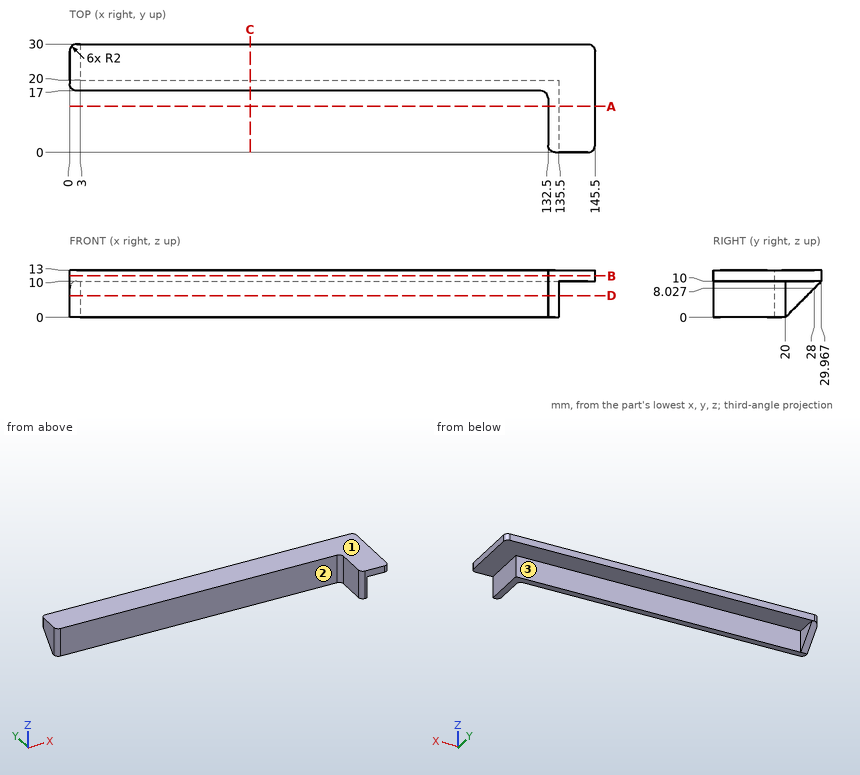
Input: dimensioned drawing with shaded views. Units: mm. Origin: part minimum x, y, z. A direction names the side the tool comes from. Round coordinates to 2 decimals unless told otherwise and drop trailing zeros. Order: outer loops, then holes, each group sorted by start corner. A loop starts at its lowest first (then second) coordinate and runs counter-clockwise, first axis right, second up. Notation, with made-up numbers: (35.5, 5.5) - (85.5, 5.5) arc R26 cw to (85.5, 44.5) - close; hole circle Ø8 at (-25, 1). An arc over 180 degrees is marked (long way). Answer as a JSON object with one key per item and string values. Group by question number.
(1) Cut plane D-D (z = 6). Return loops of the section in (x, y).
(2) Cut plane B-B (z = 11.5). Return loops of the section in (x, y).
(3) Pin query (flat end, axial travel): P1, Ø5, axis at y = 24, z = 4.5, coming from the +X side; P2, Ø4, axis at y = 12.5, z = 11, coming from the -X side; P3, Ø4, axis at x = 94.5, y = 16.5, coming from the +Z side; P4, Ø4, axis at y = 13, z = 7, coming from the +X side. Return the tip coordinate at first contact, or that it passes through.
(4) Reachability of the marked faces 1, 2 and 3 from +Z, -Z, +X, -X, +Y, -Y: full face, straight path, thin tool, end or side. Return the list, or none.
(5) Cut plane A-A (y = 12.75). Return loops of the section in (x, z).
(6) Cut plane C-C (x = 50). Return loops of the section in (y, z), then the cut area to 3 significant figures.
(7) Material intervals for probe 1 along Y at (x, z) = (69.5, 3); probe 2 along Z at (x, y) = (135.5, 20.25); probe 3 along X at (y, z) = (11.25, 7.75), sorted ascending. Write a range as from..to.
Here are the results:
{
 "1": {"outline": "(0, 19) arc R2 ccw to (2, 17) - (130.5, 17) arc R2 cw to (132.5, 15) - (132.5, 2) arc R2 ccw to (134.5, 0) - (135.5, 0) - (135.5, 20) - (3, 20) - (3, 25.98) - (0, 25.98) - close"},
 "2": {"outline": "(0, 19) arc R2 ccw to (2, 17) - (130.5, 17) arc R2 cw to (132.5, 15) - (132.5, 2) arc R2 ccw to (134.5, 0) - (143.5, 0) arc R2 ccw to (145.5, 2) - (145.5, 28) arc R2 ccw to (143.5, 30) - (2, 30) arc R2 ccw to (0, 28) - close"},
 "3": {"P1": "stops at x = 3", "P2": "stops at x = 132.5", "P3": "stops at z = 13", "P4": "stops at x = 135.5"},
 "4": {"face 1": "+Z, +X, -X, +Y, -Y", "face 2": "+Z, -Z, -X, -Y", "face 3": "-Z, +X, +Y"},
 "5": {"outline": "(132.5, 0) - (135.5, 0) - (135.5, 10) - (145.5, 10) - (145.5, 13) - (132.5, 13) - close"},
 "6": {"outline": "(17, 0) - (20, 0) - (20, 10) - (30, 10) - (30, 13) - (17, 13) - close", "area": "69.0 mm^2"},
 "7": {"probe 1": "y = 17..20", "probe 2": "z = 10..13", "probe 3": "x = 132.5..135.5"}
}
